Build history of the part. All positions in model axes, mm. A direction names the side the tool comes from. Round coordinates to 2 decimals unless told otherwise and drop trailing zeros. Order: outer loops, then holes, each group sorted by start corner. A loop starts at its lowest first (then second) coordinate and runs counter-clockwise, first axis right, second up. Notation, with made-up numbers: (67.25, 7) - (87.25, 7) arc R24 cw to (87.25, 38) - close; hole circle Ø9 at (-10.75, -1). An arc over 180 degrees is marked (long way). Write each question's results on one line, items separated by ' | '. Start each with the question number.
```python
from build123d import *

# Parameters (mm, degrees)
SKETCH1_W               = 326
SKETCH1_H               = 117.8
SKETCH1_W_2             = 318.2
SKETCH1_H_2             = 110
BOSS_EXTRUDE1_DEPTH     = 20
SKETCH1_3_W             = 318.2
SKETCH1_3_H             = 110
BOSS_EXTRUDE2_DEPTH     = 3
BOSS_EXTRUDE6_START     = 3
SKETCH6_R               = 3.25
SKETCH6_R_2             = 1.8
BOSS_EXTRUDE6_DEPTH     = 3.2
FILLET1_R               = 22
CUT_EXTRUDE3_START      = 163
CUT_EXTRUDE3_DEPTH      = 3.9
CUT_EXTRUDE4_START      = 1.2
SKETCH6_2_R             = 1.8
CUT_EXTRUDE4_DEPTH      = 1.8
SKETCH5_W               = 64.404478897
SKETCH5_H               = 11.204693833
SKETCH5_W_2             = 4
SKETCH5_H_2             = 98.795306167
SKETCH5_W_3             = 30.218685567
SKETCH5_H_3             = 8.375486052
SKETCH5_H_4             = 73.388395798
SKETCH5_W_4             = 147.589311785
SKETCH5_H_5             = 5.740206696
BOSS_EXTRUDE7_DEPTH     = 14.4
CUT_EXTRUDE5_START      = -58.9
SKETCH10_R              = 6.5
CUT_EXTRUDE5_DEPTH      = 3.9
BOSS_EXTRUDE8_START     = -55
SKETCH11_W              = 18
SKETCH11_H              = 2.429995135
SKETCH11_W_2            = 3
SKETCH11_H_2            = 3
BOSS_EXTRUDE8_DEPTH     = 3.3
BOSS_EXTRUDE9_START     = -51.7
BOSS_EXTRUDE9_DEPTH     = 3
BOSS_EXTRUDE10_START    = 3
SKETCH12_R              = 3
BOSS_EXTRUDE10_DEPTH    = 17
SKETCH12_3_R            = 3
CUT_EXTRUDE6_DEPTH      = 6
SKETCH13_R              = 4.5
CUT_EXTRUDE7_DEPTH      = 4
CUT_EXTRUDE8_DEPTH      = 30
CUT_EXTRUDE8_DEPTH_BACK = 40
SKETCH14_W              = 179.941396495
SKETCH14_H              = 132.266113534


with BuildPart() as part:
    # Sketch1 → Boss-Extrude1 (new body)
    with BuildSketch(Plane.XY):
        Rectangle(SKETCH1_W, SKETCH1_H)
        Rectangle(SKETCH1_W_2, SKETCH1_H_2, mode=Mode.SUBTRACT)
    extrude(amount=BOSS_EXTRUDE1_DEPTH)

    # Sketch1<3> → Boss-Extrude2 (add)
    with BuildSketch(Plane.XY):
        Rectangle(SKETCH1_3_W, SKETCH1_3_H)
    extrude(amount=BOSS_EXTRUDE2_DEPTH)

    # Sketch6 → Boss-Extrude6 (add)
    # profile 1 of 4: a face of its own
    with BuildSketch(Plane.XY.offset(BOSS_EXTRUDE6_START)):
        with Locations((132, -24.5)):
            Circle(SKETCH6_R)
        with Locations((132, -24.5)):
            Circle(SKETCH6_R_2, mode=Mode.SUBTRACT)
    # profile 2 of 4: a face of its own
    with BuildSketch(Plane.XY.offset(BOSS_EXTRUDE6_START)):
        with Locations((74, -24.5)):
            Circle(SKETCH6_R)
        with Locations((74, -24.5)):
            Circle(SKETCH6_R_2, mode=Mode.SUBTRACT)
    # profile 3 of 4: a face of its own
    with BuildSketch(Plane.XY.offset(BOSS_EXTRUDE6_START)):
        with Locations((74, 24.5)):
            Circle(SKETCH6_R)
        with Locations((74, 24.5)):
            Circle(SKETCH6_R_2, mode=Mode.SUBTRACT)
    # profile 4 of 4: a face of its own
    with BuildSketch(Plane.XY.offset(BOSS_EXTRUDE6_START)):
        with Locations((132, 24.5)):
            Circle(SKETCH6_R)
        with Locations((132, 24.5)):
            Circle(SKETCH6_R_2, mode=Mode.SUBTRACT)
    extrude(amount=BOSS_EXTRUDE6_DEPTH)

    # Fillet1
    fillet1_edges = [part.edges().sort_by_distance(p)[0] for p in [
        (163, 58.9, 10),
        (163, -58.9, 10),
        (-163, -58.9, 10),
        (-163, 58.9, 10),
        (159.1, 55, 11.5),
        (-159.1, 55, 11.5),
        (-159.1, -55, 11.5),
        (159.1, -55, 11.5),
    ]]
    fillet(fillet1_edges, radius=FILLET1_R)

    # Sketch9 → Cut-Extrude3 (cut)
    with BuildSketch(Plane(origin=(0, 0, 0), x_dir=(0, 0, -1), z_dir=(1, 0, 0)).offset(CUT_EXTRUDE3_START)):
        with BuildLine():
            Line((-20, -8.55), (-8.58, -8.55))
            ThreePointArc((-8.58, -8.55), (-8.226446609, -8.403553391), (-8.08, -8.05))
            Line((-8.08, -8.05), (-8.08, 6.05))
            ThreePointArc((-8.08, 6.05), (-8.226446609, 6.403553391), (-8.58, 6.55))
            Line((-8.58, 6.55), (-20, 6.55))
            Line((-20, 6.55), (-20, -8.55))
        make_face()
    extrude(amount=-CUT_EXTRUDE3_DEPTH, mode=Mode.SUBTRACT)

    # Sketch6<2> → Cut-Extrude4 (cut)
    with BuildSketch(Plane.XY.offset(CUT_EXTRUDE4_START)):
        with Locations((132, -24.5)):
            Circle(SKETCH6_2_R)
        with Locations((132, 24.5)):
            Circle(SKETCH6_2_R)
        with Locations((74, 24.5)):
            Circle(SKETCH6_2_R)
        with Locations((74, -24.5)):
            Circle(SKETCH6_2_R)
    extrude(amount=CUT_EXTRUDE4_DEPTH, mode=Mode.SUBTRACT)

    # Sketch5 → Boss-Extrude7 (add)
    with BuildSketch(Plane.XY):
        with Locations((-66.797760552, 49.397653084)):
            Rectangle(SKETCH5_W, SKETCH5_H)
        with Locations((-101, 5.602346917)):
            Rectangle(SKETCH5_W_2, SKETCH5_H_2)
        with Locations((48.890657217, 50.812256974)):
            Rectangle(SKETCH5_W_3, SKETCH5_H_3)
        with Locations((66, 49.397653084)):
            Rectangle(SKETCH5_W_2, SKETCH5_H)
        with Locations((66, 0)):
            Rectangle(SKETCH5_W_2, SKETCH5_H_4)
        with Locations((-9.794655893, -52.129896652)):
            Rectangle(SKETCH5_W_4, SKETCH5_H_5)
        with Locations((66, -49.397653084)):
            Rectangle(SKETCH5_W_2, SKETCH5_H)
    extrude(amount=BOSS_EXTRUDE7_DEPTH)

    # Sketch10 → Cut-Extrude5 (cut)
    with BuildSketch(Plane(origin=(0, 0, 0), x_dir=(1, 0, 0), z_dir=(0, 1, 0)).offset(CUT_EXTRUDE5_START)):
        with Locations((95, -16.665643961)):
            Circle(SKETCH10_R)
        with Locations((-95, -16.665643961)):
            Circle(SKETCH10_R)
    extrude(amount=CUT_EXTRUDE5_DEPTH, mode=Mode.SUBTRACT)

    # Sketch11 → Boss-Extrude8 (add)
    with BuildSketch(Plane(origin=(0, 0, 0), x_dir=(1, 0, 0), z_dir=(0, 1, 0)).offset(BOSS_EXTRUDE8_START)):
        Polygon((-104.033941149, -14.931036323), (-101.03394878, -14.937802738), (-101.040715195, -17.937795107), (-104.040707565, -17.931028692), align=None)
        Polygon((-86.018356525, -8.041657306), (-104.018310741, -8.001058815), (-104.023791526, -10.431047769), (-86.023837311, -10.47164626), align=None)
        with Locations((95, -9.450646394)):
            Rectangle(SKETCH11_W, SKETCH11_H)
        with Locations((102.5, -16.665643961)):
            Rectangle(SKETCH11_W_2, SKETCH11_H_2)
    extrude(amount=BOSS_EXTRUDE8_DEPTH)

    # Sketch11<3> → Boss-Extrude9 (add)
    with BuildSketch(Plane(origin=(0, 0, 0), x_dir=(1, 0, 0), z_dir=(0, 1, 0)).offset(BOSS_EXTRUDE9_START)):
        Polygon((86, -8.235648826), (86, -10.665643961), (91, -10.665643961), (91, -20), (99, -20), (99, -10.665643961), (104, -10.665643961), (104, -8.235648826), align=None)
        Polygon((-104.023791526, -10.431047769), (-99.023804244, -10.442325128), (-99.044857621, -19.776657424), (-91.044877969, -19.794701198), (-91.023824593, -10.460368902), (-86.023837311, -10.47164626), (-86.018356525, -8.041657306), (-104.018310741, -8.001058815), align=None)
    extrude(amount=BOSS_EXTRUDE9_DEPTH)

    # Sketch12 → Boss-Extrude10 (add)
    # profile 1 of 4: a face of its own
    with BuildSketch(Plane.XY.offset(BOSS_EXTRUDE10_START)):
        with BuildLine():
            Line((-137.1, -55), (-137.1, -48))
            ThreePointArc((-137.1, -48), (-141.493398282, -37.393398282), (-152.1, -33))
            Line((-152.1, -33), (-159.1, -33))
            ThreePointArc((-159.1, -33), (-152.656349186, -48.556349186), (-137.1, -55))
        make_face()
        with Locations((-146.828174593, -42.728174593)):
            Circle(SKETCH12_R, mode=Mode.SUBTRACT)
    # profile 2 of 4: a face of its own
    with BuildSketch(Plane.XY.offset(BOSS_EXTRUDE10_START)):
        with BuildLine():
            ThreePointArc((-137.1, 48), (-141.493398282, 37.393398282), (-152.1, 33))
            Line((-152.1, 33), (-159.1, 33))
            ThreePointArc((-159.1, 33), (-152.656349186, 48.556349186), (-137.1, 55))
            Line((-137.1, 55), (-137.1, 48))
        make_face()
        with Locations((-146.828174593, 42.728174593)):
            Circle(SKETCH12_R, mode=Mode.SUBTRACT)
    # profile 3 of 4: a face of its own
    with BuildSketch(Plane.XY.offset(BOSS_EXTRUDE10_START)):
        with BuildLine():
            ThreePointArc((152.1, 33), (141.493398282, 37.393398282), (137.1, 48))
            Line((137.1, 48), (137.1, 55))
            ThreePointArc((137.1, 55), (152.656349186, 48.556349186), (159.1, 33))
            Line((159.1, 33), (152.1, 33))
        make_face()
        with Locations((146.828174593, 42.728174593)):
            Circle(SKETCH12_R, mode=Mode.SUBTRACT)
    # profile 4 of 4: a face of its own
    with BuildSketch(Plane.XY.offset(BOSS_EXTRUDE10_START)):
        with BuildLine():
            ThreePointArc((137.1, -48), (141.493398282, -37.393398282), (152.1, -33))
            Line((152.1, -33), (159.1, -33))
            ThreePointArc((159.1, -33), (152.656349186, -48.556349186), (137.1, -55))
            Line((137.1, -55), (137.1, -48))
        make_face()
        with Locations((146.828174593, -42.728174593)):
            Circle(SKETCH12_R, mode=Mode.SUBTRACT)
    extrude(amount=BOSS_EXTRUDE10_DEPTH)

    # Sketch12<3> → Cut-Extrude6 (cut)
    with BuildSketch(Plane.XY):
        with Locations((146.828174593, 42.728174593)):
            Circle(SKETCH12_3_R)
        with Locations((146.828174593, -42.728174593)):
            Circle(SKETCH12_3_R)
        with Locations((-146.828174593, -42.728174593)):
            Circle(SKETCH12_3_R)
        with Locations((-146.828174593, 42.728174593)):
            Circle(SKETCH12_3_R)
    extrude(amount=CUT_EXTRUDE6_DEPTH, mode=Mode.SUBTRACT)

    # Sketch13 → Cut-Extrude7 (cut)
    with BuildSketch(Plane.XY):
        with Locations((-146.828174593, -42.728174593)):
            Circle(SKETCH13_R)
        with Locations((-146.828174593, 42.728174593)):
            Circle(SKETCH13_R)
        with Locations((146.828174593, 42.728174593)):
            Circle(SKETCH13_R)
        with Locations((146.828174593, -42.728174593)):
            Circle(SKETCH13_R)
    extrude(amount=CUT_EXTRUDE7_DEPTH, mode=Mode.SUBTRACT)

    # Sketch14 → Cut-Extrude8 (cut, two sides: drawn at the far end of the back side and taken through both)
    with BuildSketch(Plane.XY.offset(-CUT_EXTRUDE8_DEPTH_BACK)):
        with Locations((-89.970698248, -3.418642863)):
            Rectangle(SKETCH14_W, SKETCH14_H)
    extrude(amount=CUT_EXTRUDE8_DEPTH + CUT_EXTRUDE8_DEPTH_BACK, mode=Mode.SUBTRACT)


solid = part.part
```
1. Cut at D-D (x = 21). List the corners of the cut face in (y, z).
2. Cut at C-C (x = 81). List the corners of the cut face in (y, z), plus the area to 3 significant figures.
3. Cut at A-A (x = 50.5). List the corners of the cut face in (y, z).
4. Cut at B-B (y = -24.5). List the corners of the cut face in (x, z).
5. Flat gauge pins, fed straight in: pin 1 Ø6 at (x, y) = (32.5, -37.5) entering from -Z; pin 2 Ø3 at (x, y) = (73.5, 0.5) entering from +Z; pin 3 Ø7.5 at (x, z) = (155.5, 9) entering from -Y; pin 4 Ø3 at (x, z) = (160, 15.5) entering from -Y. Where does each tip first touch, or does it go through?
6. Mould opens along Y. For faces 4 (the face through (111, 56, 20)), 5 (the face through (150.985, -44.452, 1.972)), 6 (the face through (157, 52, 10)) say: pulls with the +Y half, pulls with the -Y half, needs draft (parallel to the pull), parting line crosses it, or undercut.
7. 3-axis set-ups, long thin cutter, end or side, ignore diameter. For faces 1 (the face through (130.2, 24.58, 3.66)), 2 (the face through (95, -52, 8.236)), 3 (the face through (150, 42, 4)): which of +Z, -Z, +X, -X, +Y, -Y reach the whole face in a straight line?
8. Wall check: line 1 (Y direction, x = 132, z = 2.5); line 2 (Y direction, x = 75.5, z = 7); line 3 (Y direction, x = 132, z = 4.55). Give the ranges that are in metal, low to high. Write a range as from..to.
A:
1) outline: (-58.9, 0) - (58.9, 0) - (58.9, 20) - (55, 20) - (55, 3) - (-49.26, 3) - (-49.26, 14.4) - (-55, 14.4) - (-55, 20) - (-58.9, 20) - close
2) outline: (-58.9, 0) - (58.9, 0) - (58.9, 20) - (55, 20) - (55, 3) - (-55, 3) - (-55, 20) - (-58.9, 20) - close | area: 486 mm^2
3) outline: (-58.9, 0) - (58.9, 0) - (58.9, 20) - (55, 20) - (55, 14.4) - (46.62, 14.4) - (46.62, 3) - (-49.26, 3) - (-49.26, 14.4) - (-55, 14.4) - (-55, 20) - (-58.9, 20) - close
4) outline: (0, 0) - (163, 0) - (163, 20) - (159.1, 20) - (159.1, 3) - (135.25, 3) - (135.25, 6.2) - (133.8, 6.2) - (133.8, 1.2) - (130.2, 1.2) - (130.2, 6.2) - (128.75, 6.2) - (128.75, 3) - (77.25, 3) - (77.25, 6.2) - (75.8, 6.2) - (75.8, 1.2) - (72.2, 1.2) - (72.2, 6.2) - (70.75, 6.2) - (70.75, 3) - (68, 3) - (68, 14.4) - (64, 14.4) - (64, 3) - (0, 3) - close
5) pin 1: stops at z = 0 | pin 2: stops at z = 3 | pin 3: stops at y = -56.09 | pin 4: stops at y = -50.23
6) face 4: needs draft | face 5: undercut | face 6: pulls with the +Y half
7) face 1: +Z | face 2: none | face 3: -Z
8) line 1: y = -58.9..-26.3, -22.7..22.7, 26.3..58.9 | line 2: y = -58.9..-55, 55..58.9 | line 3: y = -58.9..-55, -27.75..-26.3, -22.7..-21.25, 21.25..22.7, 26.3..27.75, 55..58.9
